Geometry: final body of the model. Coordinates: model frame, mm. A direction names the side the tool comes from. Round coordinates to 2 decimals unless told otherwise and drop trailing zeros. Loops run counter-clockwise (first coordinate to the right, second up) from the corner with the lowest first, then second, coordinate; pieces in that order, holes last. Notation, with made-up numbers: (81.5, 58) - (132.5, 58) arc R19 cw to (132.5, 83) - close; hole circle Ø10 at (67.25, -7). An arc over 180 degrees is marked (long way). Answer in a Markdown table with one row per item. Add a question column.
Autodesk Inventor part; units mm, degrees
ref_plane "YZ Plane" through (0, 0, 0) normal (1, 0, 0) x (0, 1, 0)
ref_plane "XZ Plane" through (0, 0, 0) normal (0, 1, 0) x (-1, 0, 0)
ref_plane "XY Plane" through (0, 0, 0) normal (0, 0, 1) x (1, 0, 0)
sketch "Skizze1" plane through (0, 0, 0) normal (1, 0, 0) x (0, 1, 0)
  line L0 (0, 0) -> (30, 0)
  line L1 (14.175552, 0) -> (14.175552, -68.187879) construction
  circle A0 centre (14.175552, -68.187879) radius 2.6
  circle A1 centre (14.175552, -68.187879) radius 7
  line L2 (0, 0) -> (7.179577, -67.95054)
  circle A2 centre (14.175552, -18.569993) radius 3.5
  arc A3 (7.675552, -4) -> (7.675552, -13) centre (7.675552, -8.5) ccw
  circle A4 centre (14.175552, -28.569993) radius 3.5
  circle A5 centre (14.175552, -38.569993) radius 3.5
  circle A6 centre (14.175552, -48.569993) radius 3.5
  circle A7 centre (14.175552, -58.569993) radius 3.5
  circle A8 centre (21.920836, -22.373144) radius 2.5
  circle A9 centre (7.389695, -22.35367) radius 2.5
  line L3 (7.675552, -4) -> (14.175552, -4)
  line L4 (7.675552, -13) -> (14.175552, -13)
  ellipse E0 centre (20.928749, -38.468301) end of major axis (19.90015, -48.968019) minor radius 0.865905
  ellipse E1 centre (7.422355, -38.468301) end of major axis (8.450954, -48.968019) minor radius 0.865905
  line L5 (21.175549, -68.194766) -> (30, 0)
  arc A10 (22.175552, -13) -> (22.175552, -4) centre (22.175552, -8.5) ccw
  line L6 (14.175552, -4) -> (22.175552, -4)
  line L7 (14.175552, -13) -> (22.175552, -13)
  point P0 (11.380257, -37.526628)
  point P1 (20.96203, -66.472155)
  dimension "d0" = 30
  dimension "d32" = 70
  dimension "d34" = 5.2
  dimension "d35" = 14
  dimension "d36" = 7
  dimension "d42" = 9
  dimension "d43" = 8.5
  dimension "d44" = 6.5
  dimension "d47" = 10
  dimension "d54" = 5
  dimension "d59" = 5
  dimension "d60" = 5
  dimension "d67" = 9
  dimension "d68" = 8
sketch "Skizze1 outline for Extrusion1" plane through (0, 0, 0) normal (1, 0, 0) x (0, 1, 0)
  circle A0 centre (14.175552, -58.569993) radius 3.5
  arc A1 (7.179577, -67.95054) -> (21.175549, -68.194766) centre (14.175552, -68.187879) ccw
  line L0 (21.175549, -68.194766) -> (30, 0)
  line L1 (30, 0) -> (0, 0)
  line L2 (0, 0) -> (7.179577, -67.95054)
  circle A2 centre (14.175552, -68.187879) radius 2.6
  arc A3 (22.175552, -13) -> (22.175552, -4) centre (22.175552, -8.5) ccw
  line L3 (22.175552, -13) -> (7.675552, -13)
  arc A4 (7.675552, -4) -> (7.675552, -13) centre (7.675552, -8.5) ccw
  line L4 (7.675552, -4) -> (22.175552, -4)
  circle A5 centre (14.175552, -48.569993) radius 3.5
  spline S0 degree 2 poles (8.450954, -48.968019) (9.9436, -48.821792) (7.654379, -33.14533) (5.365158, -17.468867) (6.161733, -33.291556) (6.958308, -49.114245) (8.450954, -48.968019) knots 0 0 0 0.33333333 0.33333333 0.66666667 0.66666667 1 1 1 weights 1 0.5 1 0.5 1 0.5 1
  circle A6 centre (14.175552, -38.569993) radius 3.5
  circle A7 centre (14.175552, -28.569993) radius 3.5
  spline S1 degree 2 poles (19.90015, -48.968019) (21.392796, -49.114245) (22.189371, -33.291556) (22.985946, -17.468867) (20.696725, -33.14533) (18.407504, -48.821792) (19.90015, -48.968019) knots 0 0 0 0.33333333 0.33333333 0.66666667 0.66666667 1 1 1 weights 1 0.5 1 0.5 1 0.5 1
  circle A8 centre (7.389695, -22.35367) radius 2.5
  circle A9 centre (14.175552, -18.569993) radius 3.5
  circle A10 centre (21.920836, -22.373144) radius 2.5
extrude "Extrusion1" add sketch "Skizze1 outline for Extrusion1" along normal blind 10
sketch "Skizze3" plane through (0, 0, 0) normal (0, 0, 1) x (1, 0, 0)
  circle A0 centre (5, 8) radius 1.7
  line L0 (0, 0) -> (10, 0)
  circle A1 centre (5, 22) radius 1.7
  line L1 (0, 30) -> (10, 30)
  line L2 (10, 30) -> (10, 0)
  dimension "d24" = 3.4
  dimension "d25" = 8
  dimension "d26" = 3.4
  dimension "d27" = 8
  dimension "d28" = 5
sketch "Skizze3 outline for Extrusion2" plane through (0, 0, 0) normal (0, 0, 1) x (1, 0, 0)
  circle A0 centre (5, 8) radius 1.7
  circle A1 centre (5, 22) radius 1.7
extrude "Extrusion2" cut sketch "Skizze3 outline for Extrusion2" against normal blind 11
chamfer "Fase1" distance 2 angle 45 1 edges at (5, 7.1796, -67.9505)
chamfer "Fase3" distance 2 angle 45 1 edges at (5, 21.1755, -68.1948)
properties part number "Radaufhängung" material "PC/ABS-Kunststoff"
1) Section B-B, the plane x = 4. Give the number of separate pieces and of enclosed holes in the cut face, and give its area (3 significant figures).
2) Contact query for flat-ended pins moving along their axis: pin 1 Ø2.5 at (x, y) = (5, 22) entering from +Z; pin 2 Ø3 at (x, z) = (2, -25.5) entering from -Y; pin 3 Ø1.5 at (x, z) = (6, -51) entering from -Y. Output: stop coordinate, or through.
3) Pull-direction query (Y, two-part tool) for faces 1 (the cylindrical face through (4.93, 13.72, -42.04)), 2 (the flat face through (4.93, 3.436, -32.519)), 3 (the flat face through (10, 18, -37)); classes: pulls with the +Y half, pulls with the -Y half, needs draft (parallel to the pull), parting line crosses it, or undercut.
4) Section C-C, the plane z = -60.5. Return the cut outline in (x, y).
5) Reachability of faces 4 (the flat face through (5, 15, -13)), 5 (the cylindrical face through (5.914, 23.433, -2.103)), 6 (the flat face through (4.93, 21.164, -68.165)) from +Z, -Z, +X, -X, +Y, -Y: full face, straight path, thin tool, end or side. Return the list, or none.
6) Material intervals for line 1 along X through (y, z) = (8, -2.5); line 2 along Y through (x, z) = (4, -45); line 3 along Z through (x, y) = (4.5, 9.5), sorted ascending. Write a range as from..to.
7) Section A-A, the plane z = -8.5. Return the cut outline in (x, y).
Evaluation:
| question | item | result |
|---|---|---|
| 1 | separate pieces | 2 |
| 1 | enclosed holes | 10 |
| 1 | area | 1,050 mm² |
| 2 | pin 1 | stops at z = -12.87 |
| 2 | pin 2 | stops at y = 2.54 |
| 2 | pin 3 | stops at y = 5.31 |
| 3 | face 1 | undercut |
| 3 | face 2 | pulls with the -Y half |
| 3 | face 3 | needs draft |
| 4 | outline | (0, 6.39) - (10, 6.39) - (10, 11.26) - (0, 11.26) - close; (0, 17.1) - (10, 17.1) - (10, 22.17) - (0, 22.17) - close |
| 5 | face 4 | +X, -X |
| 5 | face 5 | +Z |
| 5 | face 6 | -Z, +X, -X, +Y |
| 6 | line 1 | x = 0..3.3, 6.7..10 |
| 6 | line 2 | y = 4.75..7.38, 8.74..19.61, 20.97..24.18 |
| 6 | line 3 | z = -73.4..-23.69, -21.01..-13 |
| 7 | outline | (0, 0.9) - (10, 0.9) - (10, 3.18) - (0, 3.18) - close; (0, 26.68) - (10, 26.68) - (10, 28.9) - (0, 28.9) - close |
